Model file for the job. Use its own axes, mm. Face numbers are marked on the shaded views. A direction names the side the tool comes from. Coordinates: 2 decimals unless noted, no trailing zeros. Order: outer loops, then holes, each group sorted by start corner. A loop starts at its lowest first (then second) coordinate and runs counter-clockwise, first axis right, second up. Notation, with made-up numbers: (86.5, -9) -> (118.5, -9) arc R17 cw to (118.5, 7) -> close; hole circle Ø1 at (9.5, 47). An arc over 180 degrees is marked (long way). Return JSON: item names as keys, results as strings. Group by question number.
1) Which spindle directions (+Z, -Z, +X, -X, +Y, -Y) get a long thin tool onto all of the face, cutting with end or side? Do the marked faces 1 and 2. Say none if no direction does.
2) Flat gauge pins, fed straight in: pin 1 (10 mm diameter, centred on y = -31, z = -372, fed in from +X); pin 2 (5 mm diameter, centred on x = 10.5, z = -81.5, fed in from +Y); pin 3 (10 mm diameter, centred on x = -46.5, z = -524.5, fed in from -Y). Where does each tip first touch, or does it go through?
3) Cut at A-A (x = 0). Write the cut outline in (y, z).
4) Cut at C-C (z = -83). Write the cut outline in (x, y).
5) Pull direction X, two halves, no side cores. Call the marked faces 3, 4 and 5: +X half, -X half, draft (parallel to the pull), parting line (faces both ways), or undercut.
6) Probe line 1 (Y direction, x = 0, z = -638); line 2 (Z direction, x = 16, y = 117); line 3 (Z direction, x = 52, y = 30.5). List the from-to ranges inside material, lowest first.
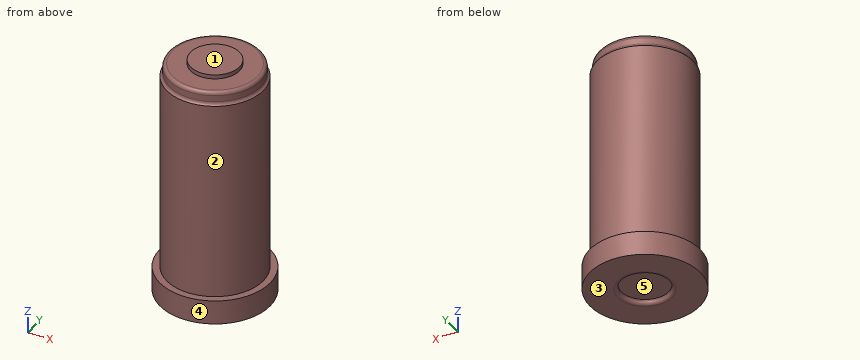
from build123d import *

# Parameters (mm, degrees)
SKETCH1_R           = 140
BOSS_EXTRUDE1_DEPTH = 580
SKETCH2_R           = 133
BOSS_EXTRUDE2_DEPTH = 38
SKETCH3_R           = 71
BOSS_EXTRUDE3_DEPTH = 12
FILLET2_R           = 10
SKETCH4_R           = 160
BOSS_EXTRUDE4_DEPTH = 70
SKETCH5_R           = 68.74
CUT_EXTRUDE1_DEPTH  = 14
FILLET3_R           = 10


with BuildPart() as part:
    # Sketch1 → Boss-Extrude1 (new body)
    with BuildSketch(Plane.XY):
        Circle(SKETCH1_R)
    extrude(amount=-BOSS_EXTRUDE1_DEPTH)

    # Sketch2 → Boss-Extrude2 (add)
    with BuildSketch(Plane.XY):
        Circle(SKETCH2_R)
    extrude(amount=BOSS_EXTRUDE2_DEPTH)

    # Sketch3 → Boss-Extrude3 (add)
    with BuildSketch(Plane.XY.offset(38)):
        Circle(SKETCH3_R)
    extrude(amount=BOSS_EXTRUDE3_DEPTH)

    # Fillet2
    # the kernel refuses this fillet: 10 mm, written as the material it adds along each edge
    with BuildSketch(Plane(origin=(0, 0, 0), x_dir=(1, 0, 0), z_dir=(0, -1, 0))) as fillet2_piece_1:
        with BuildLine():
            CenterArc((143, 9.539392014), FILLET2_R, 180, 72.542396876)
            Line((133, 9.539392014), (133, 0))
            Line((133, 0), (140, 0))
        make_face()
    revolve(axis=Axis((0, 0, 0), (0, 0, 1)))
    # the kernel refuses this fillet: 10 mm, written as the material it takes off along each edge
    with BuildSketch(Plane(origin=(0, 0, 38), x_dir=(1, 0, 0), z_dir=(0, -1, 0))) as fillet2_2_piece_1:
        with BuildLine():
            CenterArc((133 - FILLET2_R, -FILLET2_R), FILLET2_R, 0, 90)
            Line((133 - FILLET2_R, 0), (133, 0))
            Line((133, 0), (133, -FILLET2_R))
        make_face()
    revolve(axis=Axis((0, 0, 38), (0, 0, 1)), mode=Mode.SUBTRACT)

    # Sketch4 → Boss-Extrude4 (add)
    with BuildSketch(Plane(origin=(0, 0, -580), x_dir=(-1, 0, 0), z_dir=(0, 0, -1))):
        Circle(SKETCH4_R)
    extrude(amount=BOSS_EXTRUDE4_DEPTH)

    # Sketch5 → Cut-Extrude1 (cut)
    with BuildSketch(Plane(origin=(0, 0, -650), x_dir=(-1, 0, 0), z_dir=(0, 0, -1))):
        Circle(SKETCH5_R)
    extrude(amount=-CUT_EXTRUDE1_DEPTH, mode=Mode.SUBTRACT)

    # Fillet3
    fillet3_edges = [part.edges().sort_by_distance(p)[0] for p in [
        (68.74, 0, -650),
    ]]
    fillet(fillet3_edges, radius=FILLET3_R)


solid = part.part
Answers below:
{
 "1": {"face 1": "+Z, +X, -X, +Y, -Y", "face 2": "+Z"},
 "2": {"pin 1": "stops at x = 137.56", "pin 2": "stops at y = 139.77", "pin 3": "stops at y = -133.71"},
 "3": {"outline": "(-160, -650) -> (-78.74, -650) arc R10 ccw to (-68.74, -640) -> (-68.74, -636) -> (68.74, -636) -> (68.74, -640) arc R10 ccw to (78.74, -650) -> (160, -650) -> (160, -580) -> (140, -580) -> (140, 0) arc R10 cw to (133, 9.54) -> (133, 28) arc R10 ccw to (123, 38) -> (71, 38) -> (71, 50) -> (-71, 50) -> (-71, 38) -> (-123, 38) arc R10 ccw to (-133, 28) -> (-133, 9.54) arc R10 cw to (-140, 0) -> (-140, -580) -> (-160, -580) -> close"},
 "4": {"outline": "circle Ø280 at (0, 0)"},
 "5": {"face 3": "draft", "face 4": "parting line", "face 5": "undercut"},
 "6": {"line 1": "y = -160 to -68.74, 68.74 to 160", "line 2": "z = -650 to 38", "line 3": "z = -636 to 50"}
}
